Input: part model. Units: mm. Frame: model coordinates. Round coordinates to 2 decimals unless told otherwise and drop trailing zeros.
1) Section A-A, the plane x = -399.5. State how many separate pieces and enclosed holes the cut face has, and give its area (3 significant figures).
2) First-contact query: pin 1 (2 mm diameter, centred on y = -1, z = -412.5, fed in from +X); pin 2 (1.5 mm diameter, centred on y = -2, z = -624, fed in from -X); pin 3 (20.5 mm diameter, centred on x = -394.59, z = -339.07, fed in from +Y); pin 4 (2 mm diameter, centred on y = -1.5, z = -409, fed in from -X). Flat tips, straight axial feed; report the tip coordinate or a pass-through.
3) Ray query, line 1 along Z through (x, y) = (-413.5, -1.65); line 2 along X through (y, z) = (-2.5, -543); line 3 along X through (y, z) = (-3, -802). Return the intervals inside material, ascending.
4) Draft query along X for faces 1 (the face through (-395, 0, -552)), 2 (the face through (-399.373, -1.972, -634.593)). Return one class per face: pulls with the +X half, pulls with the -X half, needs draft (parallel to the pull), parting line crosses it, or undercut.
from build123d import *

# Parameters (mm, degrees)
F0_R     = 21.1586469213
F0_R_2   = 8.806010366
F0_R_3   = 12.2091210128
F0_R_4   = 17.006361888
F1_DEPTH = 4


# Not quite as in the source:
# - ends of sketch curves that miss each other by under 0.0002 mm in the source are joined


with BuildPart() as f1:
    # F0 (on Front) → F1 (new body)
    with BuildSketch(Plane.XZ):
        with BuildLine():
            Line((-404.2813370244, -555.8222100041), (-369.2932587578, -555.8222100041))
            Line((-369.2932587578, -555.8222100041), (-369.2932587578, -548.3222100041))
            Line((-369.2932587578, -548.3222100041), (-355.2932587578, -548.3222100041))
            add(Edge.make_bspline(
                [(-360.3678395822, -418.8222100041), (-357.2043853814, -459.4781491099), (-355.4697568796, -504.0564149856), (-355.2932587578, -548.3222100041)],
                knots=[0.2913303101, 0.2913303101, 0.2913303101, 0.2913303101, 0.4888396728, 0.4888396728, 0.4888396728, 0.4888396728], degree=3))
            Line((-360.3678395822, -418.8222100041), (-374.3678395822, -418.8222100041))
            Line((-374.3678395822, -418.8222100041), (-374.3678395822, -411.3222100041))
            Line((-374.3678395822, -411.3222100041), (-404.8922608862, -411.3222100041))
            Line((-404.8922608862, -411.3222100041), (-404.8922608862, -418.8222100041))
            Line((-404.8922608862, -418.8222100041), (-418.8922608862, -418.8222100041))
            add(Edge.make_bspline(
                [(-418.8922608862, -418.8222100041), (-418.5472091576, -461.9778150808), (-418.3109664436, -505.1392537968), (-418.2813370244, -548.3222100041)],
                knots=[0.2533782445, 0.2533782445, 0.2533782445, 0.2533782445, 0.4865039964, 0.4865039964, 0.4865039964, 0.4865039964], degree=3))
            Line((-418.2813370244, -548.3222100041), (-404.2813370244, -548.3222100041))
            Line((-404.2813370244, -548.3222100041), (-404.2813370244, -555.8222100041))
        make_face()
        with Locations((-387.5988423824, -520.4372406006)):
            Circle(F0_R, mode=Mode.SUBTRACT)
        with Locations((-397.4644243717, -485.6480360031)):
            Circle(F0_R_2, mode=Mode.SUBTRACT)
        with Locations((-371.7619478703, -484.8691523075)):
            Circle(F0_R_2, mode=Mode.SUBTRACT)
        with Locations((-388.8969421387, -449.0414857864)):
            Circle(F0_R, mode=Mode.SUBTRACT)
        with BuildLine():
            Line((-369.2932587578, -563.3222100041), (-369.2932587578, -555.8222100041))
            Line((-369.2932587578, -555.8222100041), (-404.2813370244, -555.8222100041))
            Line((-404.2813370244, -555.8222100041), (-404.2813370244, -563.3222100041))
            Line((-404.2813370244, -563.3222100041), (-418.2794696915, -563.3222100041))
            add(Edge.make_bspline(
                [(-418.2794696915, -563.3222100041), (-418.2983515169, -606.4848543261), (-418.524010714, -649.6671773036), (-418.8658189061, -692.8222100041)],
                knots=[0.5134952141, 0.5134952141, 0.5134952141, 0.5134952141, 0.746484428, 0.746484428, 0.746484428, 0.746484428], degree=3))
            Line((-418.8658189061, -692.8222100041), (-404.8922608862, -692.8222100041))
            Line((-404.8922608862, -692.8222100041), (-404.8922608862, -700.3222100041))
            Line((-404.8922608862, -700.3222100041), (-374.3678395822, -700.3222100041))
            Line((-374.3678395822, -700.3222100041), (-374.3678395822, -692.8222100041))
            Line((-374.3678395822, -692.8222100041), (-360.5407278397, -692.8222100041))
            add(Edge.make_bspline(
                [(-355.2933001029, -563.3222098386), (-355.473221284, -608.2616104093), (-357.267833957, -652.4575821746), (-360.5407278397, -692.8222100041)],
                knots=[0.5111757389, 0.5111757389, 0.5111757389, 0.5111757389, 0.7122386539, 0.7122386539, 0.7122386539, 0.7122386539], degree=3))
            Line((-355.2933001029, -563.3222098386), (-369.2932587578, -563.3222100041))
        make_face()
        with Locations((-388.8969421387, -662.6029342218)):
            Circle(F0_R, mode=Mode.SUBTRACT)
        with Locations((-397.4644243717, -625.9963840052)):
            Circle(F0_R_2, mode=Mode.SUBTRACT)
        with Locations((-371.7619478703, -626.7752677008)):
            Circle(F0_R_2, mode=Mode.SUBTRACT)
        with Locations((-387.5988423824, -591.2071794077)):
            Circle(F0_R, mode=Mode.SUBTRACT)
        with BuildLine():
            add(Edge.make_bspline(
                [(-361.8416139057, -707.8222100042), (-366.5966911813, -759.211500512), (-373.8431834552, -803.4077276906), (-383.2773775989, -833.5357473143)],
                knots=[0.7374547732, 0.7374547732, 0.7374547732, 0.7374547732, 1, 1, 1, 1], degree=3))
            Line((-361.8416139057, -707.8222100041), (-374.3678395822, -707.8222100041))
            Line((-374.3678395822, -707.8222100041), (-374.3678395822, -700.3222100041))
            Line((-374.3678395822, -700.3222100041), (-404.8922608862, -700.3222100041))
            Line((-404.8922608862, -700.3222100041), (-404.8922608862, -707.8222100041))
            Line((-404.8922608862, -707.8222100041), (-418.8922608862, -707.8222100041))
            Line((-418.8922608862, -707.8222100041), (-418.9891725019, -707.8222100041))
            add(Edge.make_bspline(
                [(-418.9891725019, -707.8222100041), (-419.3464745558, -749.7720501318), (-419.8036381759, -791.690950422), (-420.2773775989, -833.5357473143)],
                knots=[0.7734809807, 0.7734809807, 0.7734809807, 0.7734809807, 1, 1, 1, 1], degree=3))
            Line((-420.2773775989, -833.5357473143), (-383.2773775989, -833.5357473143))
        make_face()
        with Locations((-397.6303637028, -810.5115026041)):
            Circle(F0_R_3, mode=Mode.SUBTRACT)
        with Locations((-394.5856392384, -772.5696891352)):
            Circle(F0_R_4, mode=Mode.SUBTRACT)
        with Locations((-391.3067281246, -732.2857707544)):
            Circle(F0_R_4, mode=Mode.SUBTRACT)
        with BuildLine():
            Line((-404.8922608862, -411.3222100041), (-374.3678395822, -411.3222100041))
            Line((-374.3678395822, -411.3222100041), (-374.3678395822, -403.8222100041))
            Line((-374.3678395822, -403.8222100041), (-361.6160762359, -403.8222100041))
            add(Edge.make_bspline(
                [(-383.2773775989, -278.108672694), (-373.6927686449, -304.944377163), (-366.3661772603, -350.3256078146), (-361.6160762359, -403.8222100042)],
                knots=[0, 0, 0, 0, 0.2667311371, 0.2667311371, 0.2667311371, 0.2667311371], degree=3))
            Line((-383.2773775989, -278.108672694), (-420.2773775989, -278.108672694))
            add(Edge.make_bspline(
                [(-420.2773775989, -278.108672694), (-419.8248476428, -320.0189708532), (-419.3746825014, -361.9186969271), (-419.0164252465, -403.8222100041)],
                knots=[0, 0, 0, 0, 0.2263679612, 0.2263679612, 0.2263679612, 0.2263679612], degree=3))
            Line((-419.0164252465, -403.8222100041), (-418.8922608862, -403.8222100041))
            Line((-418.8922608862, -403.8222100041), (-404.8922608862, -403.8222100041))
            Line((-404.8922608862, -403.8222100041), (-404.8922608862, -411.3222100041))
        make_face()
        with Locations((-391.3067281246, -379.3586492538)):
            Circle(F0_R_4, mode=Mode.SUBTRACT)
        with Locations((-394.5856392384, -339.0747308731)):
            Circle(F0_R_4, mode=Mode.SUBTRACT)
        with Locations((-397.6303637028, -301.1329174042)):
            Circle(F0_R_3, mode=Mode.SUBTRACT)
    extrude(amount=F1_DEPTH)


solid = f1.part
Final values:
1. separate pieces: 13
1. enclosed holes: 0
1. area: 820 mm2
2. pin 1: stops at x = -374.37
2. pin 2: stops at x = -418.44
2. pin 3: passes through
2. pin 4: stops at x = -404.89
3. line 1: z = -833.54 to -707.82, -692.82 to -563.32, -548.32 to -418.82, -403.82 to -278.11
3. line 2: x = -418.29 to -355.32
3. line 3: x = -419.92 to -406.38, -388.88 to -375.21
4. face 1: needs draft
4. face 2: undercut
